from build123d import *

# Parameters (mm, degrees)
F0_R     = 23
F1_DEPTH = 100
F2_R     = 30
F2_R_2   = 23
F3_DEPTH = 5


with BuildPart() as f1:
    # F0 (on Top) → F1 (new body)
    with BuildSketch(Plane.XY):
        Circle(F0_R)
        with BuildLine():
            ThreePointArc((11.5, 15.124483), (0, -19), (-11.5, 15.124483))
            Line((-11.5, 15.124483), (-11.5, 11.6))
            Line((-11.5, 11.6), (11.5, 11.6))
            Line((11.5, 11.6), (11.5, 15.124483))
        make_face(mode=Mode.SUBTRACT)
    extrude(amount=F1_DEPTH)

    # F2 (on face) → F3 (join)
    with BuildSketch(Plane.XY.offset(100)):
        Circle(F2_R)
        Circle(F2_R_2, mode=Mode.SUBTRACT)
    extrude(amount=-F3_DEPTH)


solid = f1.part
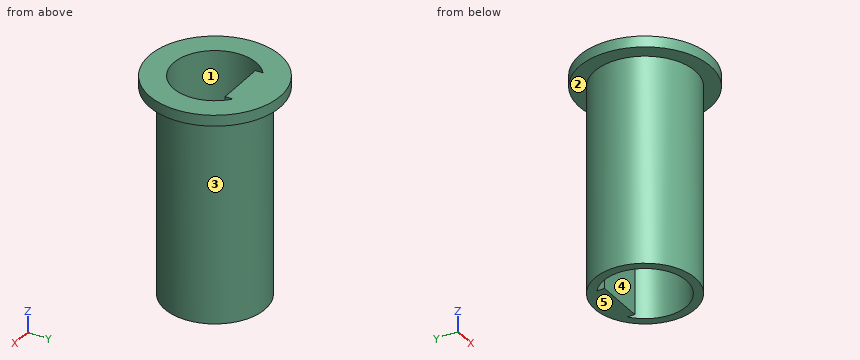
Work out the finished part from the listing and answer in its coordinate system (mm). Face numbers are marked on the shaded views. A direction names the side the tool comes from. Round coordinates to 2 decimals unless told otherwise and drop trailing zeros. Order: outer loops, then holes, each group sorted by start corner. A loop starts at its lowest first (then second) coordinate and runs counter-clockwise, first axis right, second up. Notation, with made-up numbers: M 84.25,4 L 114.25,4 A20 ccw 114.25,8 Z; hole C 24.5,-3.75 d8. An arc over 180 degrees is marked long. Put each result on its own line as item: value. Start each with the question number.
Q1. Section A-A, the plane y = 0 is taken. Write down the section's boundary in (x, z), and give its area (3 significant figures).
Q2. Flat-ended cylindrical pins translate along their axes: pin 1 (4 mm diameter, centred on y = 13.5, z = 54.5, fed in from -X); pin 2 (5 mm diameter, centred on y = 10.5, z = 43, fed in from +X); pin 3 (8 mm diameter, centred on x = 4, z = 58, fed in from -Y). Find the tip coordinate at first contact, or state that the pin passes through.
Q3. Section B-B, the plane x = 0 is taken. Write down the section's boundary in (y, z).
Q4. Section D-D, the plane y = 17.5 is taken. Write down the section's boundary in (x, z).
Q5. Section C-C, the plane z = 25.5 is taken. Write down the section's boundary in (x, y).
Q6. A tool of negligible diameter and unlimited length cuts with its end or side. For the marked faces 4 and 5, from which of +Z, -Z, +X, -X, +Y, -Y can it reach the whole face along a straight path? Write none if from no direction.
Q7. For a pull along Y with two mould halves and no side action, classify the marked faces 1, 2 and 3 as pulls with the +Y half, pulls with the -Y half, needs draft (parallel to the pull), parting line crosses it, or undercut.
Q8. Straight lines are drawn through the part: L1, parallel to X at y = 13, z = 28; L2, parallel to Y at x = 0, z = 66.5; L3, parallel to Y at x = 17, z = 18. For each, find the intervals that lie inside material, in ascending order. Write a range as [from, to].
Findings below:
1. outline: M -30,95 L -23,95 L -23,0 L -19,0 L -19,100 L -30,100 Z; M 19,0 L 23,0 L 23,95 L 30,95 L 30,100 L 19,100 Z
1. area: 870 mm^2
2. pin 1: stops at x = -19.92
2. pin 2: stops at x = 21.56
2. pin 3: stops at y = -23
3. outline: M -30,95 L -23,95 L -23,0 L -19,0 L -19,100 L -30,100 Z; M 11.6,0 L 23,0 L 23,95 L 30,95 L 30,100 L 11.6,100 Z
4. outline: M -24.37,95 L -14.92,95 L -14.92,0 L 14.92,0 L 14.92,95 L 24.37,95 L 24.37,100 L -24.37,100 Z
5. outline: C 0,0 d46; hole M -11.5,11.6 L -11.5,15.12 A19 ccw long 11.5,15.12 L 11.5,11.6 Z
6. face 4: +Z, -Z
6. face 5: -Z, +X, -X, +Y, -Y
7. face 1: undercut
7. face 2: needs draft
7. face 3: parting line crosses it
8. L1: x = [-18.97, -13.86], [-11.5, 11.5], [13.86, 18.97]
8. L2: y = [-23, -19], [11.6, 23]
8. L3: y = [-15.49, -8.49], [8.49, 15.49]
